```python
from build123d import *

# Parameters (mm, degrees)
F0_W     = 120
F0_H     = 100
F1_DEPTH = 10
F2_R     = 15
F3_DEPTH = 10.001
F4_R     = 59.99999


# Not quite as in the source:
# - a fillet or chamfer is up to 0.001 mm smaller than in the source, because OpenCascade refuses the exact size


with BuildPart() as f1:
    # F0 (on Front) → F1 (new body)
    with BuildSketch(Plane.XZ):
        Rectangle(F0_W, F0_H)
    extrude(amount=-F1_DEPTH)

    # F2 (on Front) → F3 (cut, through all)
    with BuildSketch(Plane.XZ):
        with Locations((0, -5)):
            Circle(F2_R)
    extrude(amount=-F3_DEPTH, mode=Mode.SUBTRACT)

    # F4 (radius 60 in the source; OpenCascade refuses exactly that, so slightly less here)
    f4_edges = [f1.edges().sort_by_distance(p)[0] for p in [
        (-60, 5, -50),
        (60, 5, -50),
    ]]
    fillet(f4_edges, radius=F4_R)


solid = f1.part
```
Source: CAD feature listing. Evaluate the final solid. Frame: model axes, mm. Round coordinates to 2 decimals unless told otherwise and drop trailing zeros. Order: outer loops, then holes, each group sorted by start corner. A loop starts at its lowest first (then second) coordinate and runs counter-clockwise, first axis right, second up. Notation, with made-up numbers: (44, -34) -> (62, -34) arc R25 cw to (62, -12) -> close; hole circle Ø11 at (70.25, 56.5). An arc over 180 degrees is marked (long way). Use CSV: the item, a comma, the result in double quotes.
(1) Section C-C on x = 9. Return the cut outline in (y, z), and give its area (3 significant figures).
Report:
outline,"(0, -49.32) -> (10, -49.32) -> (10, -17) -> (0, -17) -> close; (0, 7) -> (10, 7) -> (10, 50) -> (0, 50) -> close"
area,"753 mm^2"
(2) Pull-direction query (X, two-part tool) for faces 1 (the face through (-14.985, 4.93, -4.34)), 2 (the face through (-42.89, 5.07, -31.96)), 3 (the face through (-1, 0, 12)); classes: +X half, -X half, draft (parallel to the pull), parting line (faces both ways), or undercut.
Report:
face 1,"undercut"
face 2,"-X half"
face 3,"draft"
(3) Section B-B on z = -10.5. Return the cut outline in (x, y), and give its area (3 significant figures).
Report:
outline,"(-56.39, 0) -> (-13.96, 0) -> (-13.96, 10) -> (-56.39, 10) -> close; (13.96, 0) -> (56.39, 0) -> (56.39, 10) -> (13.96, 10) -> close"
area,"849 mm^2"
(4) First-contact query: pin 1 Ø3 at (y, z) = (6, 3.5) entering from -X; pin 2 Ø4 at (x, y) = (17.5, 5) entering from -Z; pin 3 Ø4 at (x, y) = (-45, 8.5) entering from -Z. Flat tips, straight axial feed; report the tip coordinate or a pass-through.
Report:
pin 1,"x = -59.79"
pin 2,"z = -47.96"
pin 3,"z = -31.84"
(5) Ray query, L1, parallel to Z at x = 5, y = 2.25; L2, parallel to Z at x = 26, y = 7; L3, parallel to X at y = 7, z = -3. Return the intervals inside material, ascending.
Report:
L1,"-49.79 to -19.14, 9.14 to 50"
L2,"-44.07 to 50"
L3,"-58.57 to -14.87, 14.87 to 58.57"
(6) Section D-D on z = -35. Return the cut outline in (x, y), and give its area (3 significant figures).
Report:
outline,"(-39.69, 0) -> (39.69, 0) -> (39.69, 10) -> (-39.69, 10) -> close"
area,"794 mm^2"
